Source: CAD feature listing. Evaluate the final solid. Frame: model axes, mm. A direction names the side the tool comes from. Round coordinates to 2 decimals unless told otherwise and drop trailing zeros. Loops run counter-clockwise (first coordinate to the right, second up) from the corner with the lowest first, then second, coordinate; pieces in that order, holes last.
Item 1: Section query A-A on y = -26. Return loops of the section in (x, z), then the cut area to 3 significant figures.
Item 2: Pull-direction query (Y, two-part tool) for faces 1 (the cylindrical face through (12.325, -35.447, 2.12)), 2 (the flat face through (0, -7, 2)), 3 (the flat face through (12, -17.6, -5)); classes: released by +Y, released by -Y, zero draft, split by the parting line, or undercut.
Item 3: Access query for faces 4 (the flat face through (12, 19, -14.15)), 5 (the cylindrical face through (0.34, -34.87, -11.75)), 6 (the cylindrical face through (24.64, -34.9, -11.73)), 7 (the flat face through (12, -17, -10.15)), 8 (the flat face through (12, 16.6, -12)). Directions: +Z, -Z, +X, -X, +Y, -Y. A direction counts if a zero-diameter tool reaches every point of the face in a straight line with its end or side. Return the directions, or none.
Item 4: First-contact query: P1, Ø2.5, axis at x = 9.5, y = -20, coming from the -Z side; P2, Ø4, axis at x = 10.5, y = 4, coming from the -Z side; P3, Ø1.1, axis at x = 7, y = -17.5, coming from the +Z side. Flat tips, straight axial feed; report the tip coordinate or a pass-through.
Item 5: Section query C-C on x = 10. Return loops of the section in (y, z) (3 decimals), then the cut area to 3 significant figures.
Item 6: Section query D-D on y = -14.5. Return loops of the section in (x, z).
Item 7: Section query B-B on z = -7. Return loops of the section in (x, y).
Item 8: Ray query, L1, parallel to Y at x = 2.75, z = -12.25 (3 decimals); L2, parallel to Z at x = 21.5, y = -29.5; L3, parallel to Z at x = 21.5, y = -17.5. Return the intervals inside material, ascending.
```python
from build123d import *

# Parameters (mm, degrees)
F1_DEPTH    = 25
F2_DEPTH    = 25
F3_T1_DEPTH = 12.2
F3_T3_DEPTH = 12.2
F3_T5_DEPTH = 12.2
F3_T7_DEPTH = 12.2
F4_T1_DEPTH = 33.6004292483


# Not quite as in the source:
# - a fillet or chamfer that OpenCascade refuses, or shapes differently, is made with other operations: its cross-section is extruded or revolved along the edge and cut away or added


with BuildPart() as f1:
    # F0 (on Right) → F1 (new body)
    with BuildSketch(Plane.YZ):
        with BuildLine():
            Line((17.6, 0.1), (17.6, -10.15))
            Line((17.6, -10.15), (16.6, -10.15))
            Line((16.6, -10.15), (16.6, -14.15))
            Line((16.6, -14.15), (21.6, -14.15))
            Line((21.6, -14.15), (21.6, 4.1))
            Line((21.6, 4.1), (0, 4.1))
            Line((0, 4.1), (-21.6, 4.1))
            Line((-21.6, 4.1), (-21.6, 1.2327951389))
            ThreePointArc((-21.6, 1.2327951389), (-19.9660188679, -1.7083752096), (-19.4, -5.025))
            ThreePointArc((-19.4, -5.025), (-19.9660188679, -8.3416247904), (-21.6, -11.2827951389))
            Line((-21.6, -11.2827951389), (-21.6, -14.15))
            Line((-21.6, -14.15), (-16.6, -14.15))
            Line((-16.6, -14.15), (-16.6, -10.15))
            Line((-16.6, -10.15), (-17.6, -10.15))
            Line((-17.6, -10.15), (-17.6, 0.1))
            Line((-17.6, 0.1), (0, 0.1))
            Line((0, 0.1), (17.6, 0.1))
        make_face()
    extrude(amount=F1_DEPTH)

    # F0 (on Right) → F2 (join)
    with BuildSketch(Plane.YZ):
        with BuildLine():
            Line((-21.6, -5.025), (-21.6, 1.2327951389))
            ThreePointArc((-21.6, 1.2327951389), (-28.8539334803, 4.9600794366), (-36.4710678119, 2.0460678119))
            Line((-36.4710678119, 2.0460678119), (-34.9154328933, 0.4904328933))
            ThreePointArc((-34.9154328933, 0.4904328933), (-26.4150692276, 2.1812603536), (-21.6, -5.025))
        make_face()
        with BuildLine():
            Line((-21.6, -11.2827951389), (-21.6, -5.025))
            ThreePointArc((-21.6, -5.025), (-26.4150692276, -12.2312603536), (-34.9154328933, -10.5404328933))
            Line((-34.9154328933, -10.5404328933), (-36.4710678119, -12.0960678119))
            ThreePointArc((-36.4710678119, -12.0960678119), (-28.8539334803, -15.0100794366), (-21.6, -11.2827951389))
        make_face()
        with BuildLine():
            ThreePointArc((-19.4, -5.025), (-19.9660188679, -1.7083752096), (-21.6, 1.2327951389))
            Line((-21.6, 1.2327951389), (-21.6, -5.025))
            Line((-21.6, -5.025), (-21.6, -11.2827951389))
            ThreePointArc((-21.6, -11.2827951389), (-19.9660188679, -8.3416247904), (-19.4, -5.025))
        make_face()
    extrude(amount=F2_DEPTH)

    # F3: fillet of radius 2 on 4 edges, made by hand

    # F3_s2 → F3_t1 (cut)
    with BuildSketch(Plane(origin=(0, -19.1923989873, -19.1923989873), x_dir=(1, 0, 0), z_dir=(0, -0.7071067812, -0.7071067812))):
        with BuildLine():
            ThreePointArc((23, 17.2357277914), (24.4142135624, 16.6499413538), (25, 15.2357277914))
            Line((25, 15.2357277914), (25, 17.2357277914))
            Line((25, 17.2357277914), (23, 17.2357277914))
        make_face()
    extrude(amount=F3_T1_DEPTH, mode=Mode.SUBTRACT)

    # F3_s4 → F3_t3 (cut)
    with BuildSketch(Plane(origin=(0, -19.1923989873, -19.1923989873), x_dir=(1, 0, 0), z_dir=(0, -0.7071067812, -0.7071067812))):
        with BuildLine():
            ThreePointArc((0, 15.2357277914), (0.5857864376, 16.6499413538), (2, 17.2357277914))
            Line((2, 17.2357277914), (0, 17.2357277914))
            Line((0, 17.2357277914), (0, 15.2357277914))
        make_face()
    extrude(amount=F3_T3_DEPTH, mode=Mode.SUBTRACT)

    # F3_s6 → F3_t5 (cut)
    with BuildSketch(Plane(origin=(0, -22.7941017178, 22.7941017178), x_dir=(1, 0, 0), z_dir=(0, 0.7071067812, -0.7071067812))):
        with BuildLine():
            ThreePointArc((25, 22.3421509423), (24.4142135624, 23.7563645047), (23, 24.3421509423))
            Line((23, 24.3421509423), (25, 24.3421509423))
            Line((25, 24.3421509423), (25, 22.3421509423))
        make_face()
    extrude(amount=F3_T5_DEPTH, mode=Mode.SUBTRACT)

    # F3_s8 → F3_t7 (cut)
    with BuildSketch(Plane(origin=(0, -22.7941017178, 22.7941017178), x_dir=(1, 0, 0), z_dir=(0, 0.7071067812, -0.7071067812))):
        with BuildLine():
            ThreePointArc((0, 22.3421509423), (0.5857864376, 23.7563645047), (2, 24.3421509423))
            Line((2, 24.3421509423), (0, 24.3421509423))
            Line((0, 24.3421509423), (0, 22.3421509423))
        make_face()
    extrude(amount=F3_T7_DEPTH, mode=Mode.SUBTRACT)

    # F4: fillet of radius 2 on 2 edges, made by hand

    # F4_s2 → F4_t1 (cut)
    with BuildSketch(Plane.YZ.offset(-4.3002146241)):
        with BuildLine():
            ThreePointArc((-34.8772255751, 0.4522255751), (-35.4470714052, 2.1184477224), (-34.4787650158, 3.5892989218))
            ThreePointArc((-34.4787650158, 3.5892989218), (-35.523724357, 2.8806941504), (-36.4710678119, 2.0460678119))
            Line((-36.4710678119, 2.0460678119), (-34.8772255751, 0.4522255751))
        make_face()
        with BuildLine():
            ThreePointArc((-34.8772255751, -10.5022255751), (-35.4470714052, -12.1684477224), (-34.4787650158, -13.6392989218))
            ThreePointArc((-34.4787650158, -13.6392989218), (-35.523724357, -12.9306941504), (-36.4710678119, -12.0960678119))
            Line((-36.4710678119, -12.0960678119), (-34.8772255751, -10.5022255751))
        make_face()
    extrude(amount=F4_T1_DEPTH, mode=Mode.SUBTRACT)


solid = f1.part
```
Data:
1. outline: (0, -14.43) - (25, -14.43) - (25, -12.04) - (0, -12.04) - close; (0, 1.99) - (25, 1.99) - (25, 4.38) - (0, 4.38) - close
1. area: 119 mm2
2. face 1: released by -Y
2. face 2: zero draft
2. face 3: undercut
3. face 4: -Z, +X, -X, +Y
3. face 5: -X, -Y
3. face 6: +X, -Y
3. face 7: +X, -X
3. face 8: -Z, +X, -X
4. P1: stops at z = -14.15
4. P2: stops at z = 0.1
4. P3: stops at z = 4.1
5. outline: (-34.915, -10.541) arc R2 ccw to (-34.479, -13.639) arc R10 ccw to (-21.6, -11.283) - (-21.6, -14.15) - (-16.6, -14.15) - (-16.6, -10.15) - (-17.6, -10.15) - (-17.6, 0.1) - (17.6, 0.1) - (17.6, -10.15) - (16.6, -10.15) - (16.6, -14.15) - (21.6, -14.15) - (21.6, 4.1) - (-21.6, 4.1) - (-21.6, 1.233) arc R10 ccw to (-34.479, 3.589) arc R2 ccw to (-34.915, 0.491) arc R7.8 cw (long way) to start
5. area: 366 mm2
6. outline: (0, 0.1) - (25, 0.1) - (25, 4.1) - (0, 4.1) - close
7. outline: (0, -21.85) - (25, -21.85) - (25, -17.6) - (0, -17.6) - close; (0, 17.6) - (25, 17.6) - (25, 21.6) - (0, 21.6) - close
8. L1: y = -35.435 to -32.339, -26.461 to -22.486, -21.6 to -16.6, 16.6 to 21.6
8. L2: z = -15.02 to -12.82, 2.77 to 4.97
8. L3: z = -14.15 to -10.15, 0.1 to 4.1
